from build123d import *

# Parameters (mm, degrees)
SKETCH2_R           = 6
SKETCH2_R_2         = 1.5
BOSS_EXTRUDE1_DEPTH = 1.15
SKETCH3_R           = 4.4
BOSS_EXTRUDE2_DEPTH = 3.2
SKETCH4_R           = 0.75
BOSS_EXTRUDE3_DEPTH = 1.15
CIRPATTERN1_COUNT   = 6


with BuildPart() as part:
    # Sketch2 → Boss-Extrude1 (new, symmetric)
    with BuildSketch(Plane(origin=(0, 0, 0), x_dir=(1, 0, 0), z_dir=(0, 1, 0))):
        with Locations(Location((0, 0, 0), (0, 0, 270))):
            Circle(SKETCH2_R)
        with Locations(Location((0, 0, 0), (0, 0, 270))):
            Circle(SKETCH2_R_2, mode=Mode.SUBTRACT)
    extrude(amount=BOSS_EXTRUDE1_DEPTH, both=True)

    # Sketch3 → Boss-Extrude2 (add)
    with BuildSketch(Plane(origin=(0, 1.15, 0), x_dir=(1, 0, 0), z_dir=(0, 1, 0))):
        with Locations(Location((0, 0, 0), (0, 0, 270))):
            Circle(SKETCH3_R)
        with BuildLine():
            Line((0.107421435, 2.898009771), (0.338399731, 2.678709694))
            Line((0.338399731, 2.678709694), (0.61665913, 2.83367809))
            ThreePointArc((0.61665913, 2.83367809), (0.721200673, 2.808891167), (0.824752316, 2.780248841))
            Line((0.824752316, 2.780248841), (0.993936292, 2.510396512))
            Line((0.993936292, 2.510396512), (1.301992734, 2.591295993))
            ThreePointArc((1.301992734, 2.591295993), (1.397085655, 2.541289372), (1.490260976, 2.48779465))
            Line((1.490260976, 2.48779465), (1.587020181, 2.184345885))
            Line((1.587020181, 2.184345885), (1.905517346, 2.186093238))
            ThreePointArc((1.905517346, 2.186093238), (1.985186607, 2.11400902), (2.062131058, 2.039023173))
            Line((2.062131058, 2.039023173), (2.080385755, 1.721044772))
            Line((2.080385755, 1.721044772), (2.389311295, 1.643530205))
            ThreePointArc((2.389311295, 1.643530205), (2.448550984, 1.553897705), (2.504429862, 1.46213237))
            Line((2.504429862, 1.46213237), (2.443033042, 1.149604087))
            Line((2.443033042, 1.149604087), (2.722976028, 0.997698125))
            ThreePointArc((2.722976028, 0.997698125), (2.758063897, 0.896149284), (2.789366126, 0.793370413))
            Line((2.789366126, 0.793370413), (2.652175577, 0.505929549))
            Line((2.652175577, 0.505929549), (2.885546163, 0.289177003))
            ThreePointArc((2.885546163, 0.289177003), (2.894277512, 0.182092507), (2.899036259, 0.074758075))
            Line((2.899036259, 0.074758075), (2.694672167, -0.169534403))
            Line((2.694672167, -0.169534403), (2.866806821, -0.437514174))
            ThreePointArc((2.866806821, -0.437514174), (2.848633027, -0.543405812), (2.826549281, -0.648551587))
            Line((2.826549281, -0.648551587), (2.567852594, -0.834345885))
            Line((2.567852594, -0.834345885), (2.667935462, -1.136714727))
            ThreePointArc((2.667935462, -1.136714727), (2.623998452, -1.234759946), (2.576459817, -1.331110368))
            Line((2.576459817, -1.331110368), (2.279685399, -1.446732346))
            Line((2.279685399, -1.446732346), (2.301427906, -1.764491312))
            ThreePointArc((2.301427906, -1.764491312), (2.234488404, -1.84852957), (2.164481907, -1.930030589))
            Line((2.164481907, -1.930030589), (1.848277186, -1.968215294))
            Line((1.848277186, -1.968215294), (1.790313171, -2.281398419))
            ThreePointArc((1.790313171, -2.281398419), (1.704577232, -2.346149284), (1.616501638, -2.40767989))
            Line((1.616501638, -2.40767989), (1.30073492, -2.366028036))
            Line((1.30073492, -2.366028036), (1.166706475, -2.654956874))
            ThreePointArc((1.166706475, -2.654956874), (1.067561203, -2.696351809), (0.966950626, -2.734045809))
            Line((0.966950626, -2.734045809), (0.671462695, -2.615174535))
            Line((0.671462695, -2.615174535), (0.469791321, -2.861694623))
            ThreePointArc((0.469791321, -2.861694623), (0.363466377, -2.877132634), (0.25664255, -2.888621575))
            Line((0.25664255, -2.888621575), (0, -2.7))
            Line((0, -2.7), (-0.25664255, -2.888621575))
            ThreePointArc((-0.25664255, -2.888621575), (-0.363466377, -2.877132634), (-0.469791321, -2.861694623))
            Line((-0.469791321, -2.861694623), (-0.671462695, -2.615174535))
            Line((-0.671462695, -2.615174535), (-0.966950626, -2.734045809))
            ThreePointArc((-0.966950626, -2.734045809), (-1.067561203, -2.696351809), (-1.166706475, -2.654956874))
            Line((-1.166706475, -2.654956874), (-1.30073492, -2.366028036))
            Line((-1.30073492, -2.366028036), (-1.616501638, -2.40767989))
            ThreePointArc((-1.616501638, -2.40767989), (-1.704577232, -2.346149284), (-1.790313171, -2.281398419))
            Line((-1.790313171, -2.281398419), (-1.848277186, -1.968215294))
            Line((-1.848277186, -1.968215294), (-2.164481907, -1.930030589))
            ThreePointArc((-2.164481907, -1.930030589), (-2.234488404, -1.84852957), (-2.301427906, -1.764491312))
            Line((-2.301427906, -1.764491312), (-2.279685399, -1.446732346))
            Line((-2.279685399, -1.446732346), (-2.576459817, -1.331110368))
            ThreePointArc((-2.576459817, -1.331110368), (-2.623998452, -1.234759946), (-2.667935462, -1.136714727))
            Line((-2.667935462, -1.136714727), (-2.567852594, -0.834345885))
            Line((-2.567852594, -0.834345885), (-2.826549281, -0.648551587))
            ThreePointArc((-2.826549281, -0.648551587), (-2.848633027, -0.543405812), (-2.866806821, -0.437514174))
            Line((-2.866806821, -0.437514174), (-2.694672167, -0.169534403))
            Line((-2.694672167, -0.169534403), (-2.899036259, 0.074758075))
            ThreePointArc((-2.899036259, 0.074758075), (-2.894277512, 0.182092507), (-2.885546163, 0.289177003))
            Line((-2.885546163, 0.289177003), (-2.652175577, 0.505929549))
            Line((-2.652175577, 0.505929549), (-2.789366126, 0.793370413))
            ThreePointArc((-2.789366126, 0.793370413), (-2.758063897, 0.896149284), (-2.722976028, 0.997698125))
            Line((-2.722976028, 0.997698125), (-2.443033042, 1.149604087))
            Line((-2.443033042, 1.149604087), (-2.504429862, 1.46213237))
            ThreePointArc((-2.504429862, 1.46213237), (-2.448550984, 1.553897705), (-2.389311295, 1.643530205))
            Line((-2.389311295, 1.643530205), (-2.080385755, 1.721044772))
            Line((-2.080385755, 1.721044772), (-2.062131058, 2.039023173))
            ThreePointArc((-2.062131058, 2.039023173), (-1.985186607, 2.11400902), (-1.905517346, 2.186093238))
            Line((-1.905517346, 2.186093238), (-1.587020181, 2.184345885))
            Line((-1.587020181, 2.184345885), (-1.490260976, 2.48779465))
            ThreePointArc((-1.490260976, 2.48779465), (-1.397085655, 2.541289372), (-1.301992734, 2.591295993))
            Line((-1.301992734, 2.591295993), (-0.993936292, 2.510396512))
            Line((-0.993936292, 2.510396512), (-0.824752316, 2.780248841))
            ThreePointArc((-0.824752316, 2.780248841), (-0.721200673, 2.808891167), (-0.61665913, 2.83367809))
            Line((-0.61665913, 2.83367809), (-0.338399731, 2.678709694))
            Line((-0.338399731, 2.678709694), (-0.107421435, 2.898009771))
            ThreePointArc((-0.107421435, 2.898009771), (0, 2.9), (0.107421435, 2.898009771))
        make_face(mode=Mode.SUBTRACT)
    extrude(amount=BOSS_EXTRUDE2_DEPTH)

    # Sketch4 → Boss-Extrude3 (add, symmetric)
    with BuildSketch(Plane(origin=(0, 0, 0), x_dir=(1, 0, 0), z_dir=(0, 1, 0))):
        with BuildLine():
            Line((3.968626967, 4.5), (14.000671478, 2.449352582))
            ThreePointArc((14.000671478, 2.449352582), (16, 0), (14.000671478, -2.449352582))
            Line((14.000671478, -2.449352582), (3.968626967, -4.5))
            ThreePointArc((3.968626967, -4.5), (6, 0), (3.968626967, 4.5))
        make_face()
        with Locations(Location((13, 0, 0), (0, 0, 270))):
            Circle(SKETCH4_R, mode=Mode.SUBTRACT)
        with Locations(Location((10, 0, 0), (0, 0, 270))):
            Circle(SKETCH4_R, mode=Mode.SUBTRACT)
        with Locations(Location((7, 0, 0), (0, 0, 270))):
            Circle(SKETCH4_R, mode=Mode.SUBTRACT)
    boss_extrude3 = extrude(amount=BOSS_EXTRUDE3_DEPTH, both=True)

    # CirPattern1: Boss-Extrude3 ×6 about axis
    cirpattern1_axis = Axis((0, 0, 0), (0, 1, 0))
    for i in range(1, CIRPATTERN1_COUNT):
        add(boss_extrude3.rotate(cirpattern1_axis, i * 360 / CIRPATTERN1_COUNT))


solid = part.part
For this review, take the finished solid that the model builds, in its own axes (mm). A direction names the side the tool comes from. Round coordinates to 2 decimals unless told otherwise and drop trailing zeros. Order: outer loops, then holes, each group sorted by start corner. A loop starts at its lowest first (then second) coordinate and runs counter-clockwise, first axis right, second up. Notation, with made-up numbers: (79.5, -20) -> (83.5, -20) arc R19 cw to (83.5, -13) -> close; hole circle Ø5 at (70.25, 71). An arc over 180 degrees is marked (long way). Write item = value, one per line. Start each with the question number.
1) Take a section at C-C on y = -0.25. Count the separate pieces of the cut face and the enclosed holes in it, plus the area to 3 significant figures.
2) Insertion check: pin 1 (2 mm diameter, centred on x = -8.5, y = 0, fed in from -Z); pin 2 (1.7 mm diameter, centred on x = -13, z = 0, fed in from +Y); pin 3 (1.5 mm diameter, centred on y = 2.5, z = -3, fed in from -X). Each pin has a flat end and moves straight along its axis. Give the tip position at first contact, or say it passes through.
3) Tool access review of faces 1 (the face through (10.347, 0.016, -3.196)), 2 (the face through (-6.71, -0.02, -0.69)), 3 (the face through (-2.474, 0.016, -10.636)): name each direction out of +Z, -Z, +X, -X, +Y, -Y from which nothing blocks a thin tool from reaching the whole face with its end or side.
4) Take a section at D-D on z = -7.25. State the section outline as (x, y) points, plus the area to 3 significant figures.
5) Take a section at A-A on x = -13. State the section outline as (y, z) points, plus the area to 3 significant figures.
6) The part is to be moulded in two halves that separate along Z. For faces 4 (the face through (-2.405, 0.016, 10.559)), 5 (the face through (-16, 0, 0)), 6 (the face through (-10.744, -0.016, 0.098)), say which applies: +Z half, -Z half, draft (parallel to the pull), parting line (faces both ways), or undercut.
7) Take a section at B-B on x = -3.5. State the section outline as (y, z) points.
8) To check wall thickness, follow line 1 (X direction, y = -0.2, z = 6.5); line 2 (Z direction, x = 3, y = 1.1); line 3 (X direction, y = -0.1, z = -11.25). State the ranges of each line that lie inside material, in increasing order. Write a range as from..to.
Verdict:
q1.separate_pieces = 1
q1.enclosed_holes = 19
q1.area = 441 mm2
q2.pin_1 = -14.08
q2.pin_2 = 1.15
q2.pin_3 = -3.78
q3.face_1 = +X, +Y, -Y
q3.face_2 = +Y, -Y
q3.face_3 = -Z, +Y, -Y
q4.outline = (-7.9, -1.15) -> (7.9, -1.15) -> (7.9, 1.15) -> (-7.9, 1.15) -> close
q4.area = 36.4 mm2
q5.outline = (-1.15, -2.65) -> (1.15, -2.65) -> (1.15, -0.75) -> (-1.15, -0.75) -> close; (-1.15, 0.75) -> (1.15, 0.75) -> (1.15, 2.65) -> (-1.15, 2.65) -> close
q5.area = 8.76 mm2
q6.face_4 = +Z half
q6.face_5 = parting line
q6.face_6 = undercut
q7.outline = (-1.15, -11.79) -> (1.15, -11.79) -> (1.15, -6.81) -> (-1.15, -6.81) -> close; (-1.15, -5.31) -> (1.15, -5.31) -> (1.15, -2.67) -> (4.35, -2.67) -> (4.35, 2.67) -> (1.15, 2.67) -> (1.15, 5.31) -> (-1.15, 5.31) -> close; (-1.15, 6.81) -> (1.15, 6.81) -> (1.15, 11.79) -> (-1.15, 11.79) -> close
q8.line_1 = -7.65..-4.11, -2.89..2.89, 4.11..7.65
q8.line_2 = -11.23..-6.62, -5.5..5.5, 6.62..11.23
q8.line_3 = -9.21..-7.25, -5.75..-3.02, 3.02..5.75, 7.25..9.21
